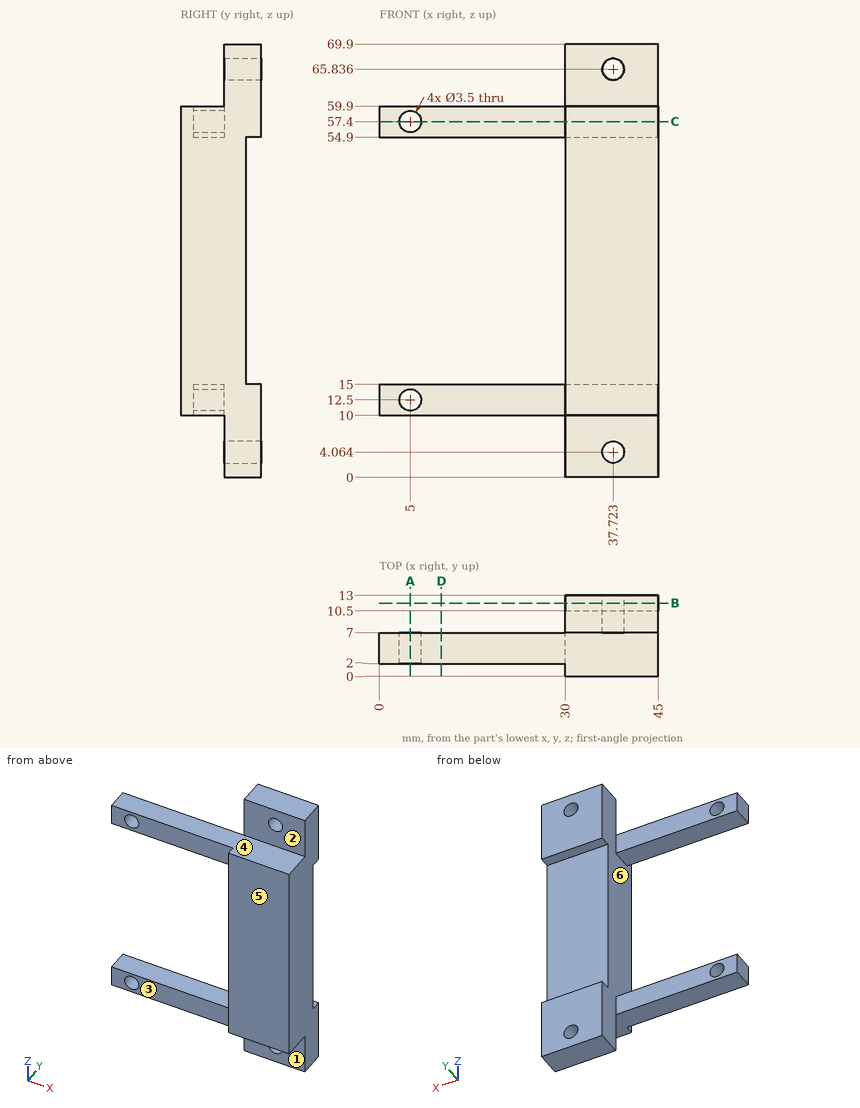
Answer from the drawing. Dimensions are ordinates in mm from the lowest x, y and z of the part. A direction names the side the tool comes from. Round coordinates to 2 decimals unless told otherwise and drop trailing zeros. Loops run counter-clockwise (first coordinate to the right, second up) from the corner with the lowest first, then second, coordinate; pieces in that order, holes last.
Q1. Section B-B on y = 11.75 is taken. Give the number of separate pieces and of enclosed holes in the cut face, and give its area (3 significant figures).
Q2. Determine the mould class of the marked faces 4, 5 and 6 for opening direction Z: released by +Z, released by -Z, zero draft, split by the parting line, or undercut.
Q3. Consider probe 1 along X at (y, z) = (2.5, 57.5); probe 2 along Z at (x, y) = (8, 2.25); probe 3 along Z at (x, y) = (38.5, 7.75) (1 decimal). Determine where each line is inside the solid, lowest interval first.
Q4. Each of these flat-tipped pins is pushed along its axis until it touches: pin 1 (4 mm diameter, centred on x = 18.5, z = 57.5, fed in from -Y); pin 2 (2.5 mm diameter, centred on x = 21, y = 3.5, fed in from -Z); pin 3 (4 mm diameter, centred on x = 5, z = 12.5, fed in from +Y). Where does it stop, or does it pass through?
Q5. Section D-D on x = 10 is taken. Write down the section's boundary in (y, z), and give its area (3 significant figures).
Q6. Which of the six approach directions +Z, -Z, +X, -X, +Y, -Y give full straight-line access (tool end or side, diameter ignored) to the marked faces 1, 2 and 3?
Q7. Section A-A on x = 5 is taken. Write down the section's boundary in (y, z).
Q8. Section C-C on z = 57.4 is taken. Write down the section's boundary in (x, y).
Output:
1. separate pieces: 2
1. enclosed holes: 2
1. area: 431 mm2
2. face 4: released by +Z
2. face 5: zero draft
2. face 6: undercut
3. probe 1: x = 0 to 3.25, 6.75 to 45
3. probe 2: z = 10 to 15, 54.9 to 59.9
3. probe 3: z = 0 to 2.5, 5.6 to 64.3, 67.4 to 69.9
4. pin 1: stops at y = 2
4. pin 2: stops at z = 10
4. pin 3: stops at y = 7
5. outline: (2, 10) - (7, 10) - (7, 15) - (2, 15) - close; (2, 54.9) - (7, 54.9) - (7, 59.9) - (2, 59.9) - close
5. area: 50.0 mm2
6. face 1: -Z, +X, -X, -Y
6. face 2: +Z, +X, -X, -Y
6. face 3: +Z, -Z, -X, -Y
7. outline: (2, 10) - (7, 10) - (7, 10.75) - (2, 10.75) - close; (2, 14.25) - (7, 14.25) - (7, 15) - (2, 15) - close; (2, 54.9) - (7, 54.9) - (7, 55.65) - (2, 55.65) - close; (2, 59.15) - (7, 59.15) - (7, 59.9) - (2, 59.9) - close
8. outline: (0, 2) - (3.25, 2) - (3.25, 7) - (0, 7) - close; (6.75, 2) - (30, 2) - (30, 0) - (45, 0) - (45, 13) - (30, 13) - (30, 7) - (6.75, 7) - close
